Could you check a few things on this drawing? It's one solid part, dimensions in mm from its lowest x, y, z. A direction names the side the tool comes from. Give positions to 0.01 mm unless a question says otherwise; leave off trailing zeros. Order: outer loops, then holes, each group sorted by start corner. A loop starts at its lowest first (then second) coordinate and runs counter-clockwise, first axis right, second up. Notation, with made-up numbers: M -29.5,63 L 9.5,63 A32 ccw 9.5,98 Z; hole C 65.25,-5.5 d11. An arc over 180 degrees is marked long. Use one line per item in the form item = value.
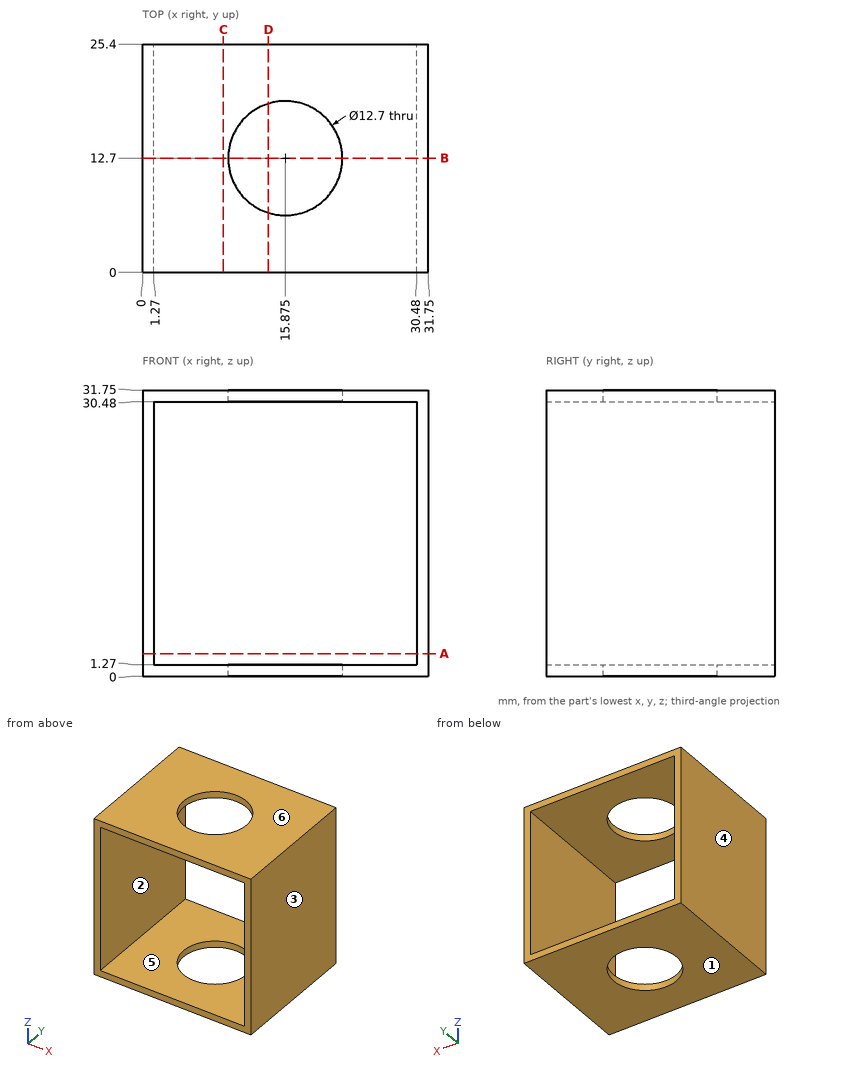
Q1. I need wall thicknesses on L1, parallel to Z at x = 10, y = 4. Which ranges of the line are inside material? Lowest first, please.
Found:
L1 = 0 to 1.27, 30.48 to 31.75
Q2. I want a section at B-B on y = 12.7. Write out the boundary of the cut face in (x, z) (3 decimals), then the cut area to 3 significant figures.
Found:
outline = M 0,0 L 9.525,0 L 9.525,1.27 L 1.27,1.27 L 1.27,30.48 L 9.525,30.48 L 9.525,31.75 L 0,31.75 Z; M 22.225,0 L 31.75,0 L 31.75,31.75 L 22.225,31.75 L 22.225,30.48 L 30.48,30.48 L 30.48,1.27 L 22.225,1.27 Z
area = 123 mm²
Q3. On a 3-axis mill with a long thin cutter (end or side, diameter ignored), from which of +Z, -Z, +X, -X, +Y, -Y can I reach the whole of each face in a straight line? I mean the marked faces 1 and 2. Say none if no direction works.
Found:
face_1 = -Z, +X, -X, +Y, -Y
face_2 = +Y, -Y
Q4. I want a section at A-A on z = 2.5. Write out the boundary of the cut face in (x, y).
Found:
outline = M 0,0 L 1.27,0 L 1.27,25.4 L 0,25.4 Z; M 30.48,0 L 31.75,0 L 31.75,25.4 L 30.48,25.4 Z
Q5. I want a section at D-D on x = 14. Write out the boundary of the cut face in (y, z), then the cut area to 3 significant figures.
Found:
outline = M 0,0 L 6.63,0 L 6.63,1.27 L 0,1.27 Z; M 0,30.48 L 6.63,30.48 L 6.63,31.75 L 0,31.75 Z; M 18.77,0 L 25.4,0 L 25.4,1.27 L 18.77,1.27 Z; M 18.77,30.48 L 25.4,30.48 L 25.4,31.75 L 18.77,31.75 Z
area = 33.7 mm²
Q6. I want a section at C-C on x = 9. Write out the boundary of the cut face in (y, z).
Found:
outline = M 0,0 L 25.4,0 L 25.4,1.27 L 0,1.27 Z; M 0,30.48 L 25.4,30.48 L 25.4,31.75 L 0,31.75 Z
Q7. Thinking about a two-plate mould opening in X: for the marked faces 3, 4, 5 and 6, which applies, +X half, -X half, draft (parallel to the pull), parting line (faces both ways), or undercut?
Found:
face_3 = +X half
face_4 = -X half
face_5 = undercut
face_6 = draft
